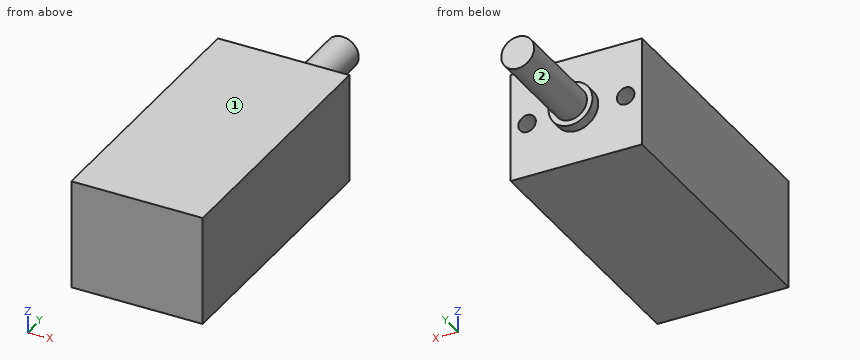
from build123d import *

# Parameters (mm, degrees)
SKETCH_1_W          = 12
SKETCH_1_H          = 10
EXTRUDE_1_DEPTH     = 25
SKETCH_2_R          = 2
EXTRUDE_2_DEPTH     = 1
SKETCH_3_R          = 1.5
EXTRUDE_3_DEPTH     = 9
SKETCH_4_R          = 0.8
CUT_EXTRUDE_1_DEPTH = 5


with BuildPart() as part:
    # 草图1 → 凸台-拉伸1 (new body)
    with BuildSketch(Plane(origin=(0, 0, 0), x_dir=(1, 0, 0), z_dir=(0, 1, 0))):
        Rectangle(SKETCH_1_W, SKETCH_1_H)
    extrude(amount=EXTRUDE_1_DEPTH)

    # 草图2 → 凸台-拉伸2 (add)
    with BuildSketch(Plane(origin=(0, 25, 0), x_dir=(1, 0, 0), z_dir=(0, 1, 0))):
        with Locations(Location((0, 0, 0), (0, 0, 270))):
            Circle(SKETCH_2_R)
    extrude(amount=EXTRUDE_2_DEPTH)

    # 草图3 → 凸台-拉伸3 (add)
    with BuildSketch(Plane(origin=(0, 26, 0), x_dir=(1, 0, 0), z_dir=(0, 1, 0))):
        with Locations(Location((0, 0, 0), (0, 0, 270))):
            Circle(SKETCH_3_R)
    extrude(amount=EXTRUDE_3_DEPTH)

    # 草图4 → 切除-拉伸1 (cut)
    with BuildSketch(Plane(origin=(0, 25, 0), x_dir=(1, 0, 0), z_dir=(0, 1, 0))):
        with Locations(Location((-4.5, 0, 0), (0, 0, 270))):
            Circle(SKETCH_4_R)
        with Locations(Location((4.5, 0, 0), (0, 0, 270))):
            Circle(SKETCH_4_R)
    extrude(amount=-CUT_EXTRUDE_1_DEPTH, mode=Mode.SUBTRACT)


solid = part.part
Can you work these out from the model? Positions are in its coordinate system, mm. Face numbers are marked on the shaded views. A direction names the side the tool comes from. Coordinates: 2 decimals unless noted, no trailing zeros. Write each loop counter-clockwise with the first axis right and the second up, starting at its lowest first coordinate (ties: lowest second). Pieces come first, ordered by that corner, then holes. Notation, with made-up numbers: (44.25, 70) - (56.25, 70) arc R22 cw to (56.25, 80) - close; hole circle Ø3 at (36, 34.5). An arc over 180 degrees is marked (long way). Return JSON: item names as keys, results as strings. Group by question number.
Item 1: If we section it at A-A (y = 20.5): Write out the boundary of the cut face in (x, z).
Item 2: I'm going to push flat-ended pins straight in: pin 1 Ø2 at (x, z) = (3.5, -2) entering from +Y; pin 2 Ø5 at (y, z) = (30, 1.5) entering from +X; pin 3 Ø0.8 at (x, z) = (-4.5, 0) entering from +Y. Where does each tip first touch, or does it pass through?
Item 3: Which directions (+Z, -Z, +X, -X, +Y, -Y) give clear straight access to the entire face, cutting with the end or side of a thin tool? Please do the marked faces 1 and 2.
Item 4: If we section it at D-D (y = 29.5): Write out the boundary of the cut face in (x, z), then the cut area to 3 significant figures.
Item 5: If we section it at B-B (x = 0): Write out the boundary of the cut face in (y, z), then the cut area to 3 significant figures.
Item 6: If we section it at C-C (z = 0): Write out the boundary of the cut face in (x, y), then the cut area to 3 significant figures.
Item 7: Please list where these lines run through material, in increasing order: probe 1 along X at (y, z) = (23.9, 0); probe 2 along Y at (x, z) = (4.25, 3.5); probe 3 along Y at (x, z) = (-4, 0.25).
Return value:
{
 "1": {"outline": "(-6, -5) - (6, -5) - (6, 5) - (-6, 5) - close; hole circle Ø1.6 at (-4.5, 0); hole circle Ø1.6 at (4.5, 0)"},
 "2": {"pin 1": "stops at y = 25", "pin 2": "stops at x = 1.5", "pin 3": "stops at y = 20"},
 "3": {"face 1": "+Z, +X, -X, +Y, -Y", "face 2": "+Y"},
 "4": {"outline": "circle Ø3 at (0, 0)", "area": "7.07 mm^2"},
 "5": {"outline": "(0, -5) - (25, -5) - (25, -2) - (26, -2) - (26, -1.5) - (35, -1.5) - (35, 1.5) - (26, 1.5) - (26, 2) - (25, 2) - (25, 5) - (0, 5) - close", "area": "281 mm^2"},
 "6": {"outline": "(-6, 0) - (6, 0) - (6, 25) - (5.3, 25) - (5.3, 20) - (3.7, 20) - (3.7, 25) - (2, 25) - (2, 26) - (1.5, 26) - (1.5, 35) - (-1.5, 35) - (-1.5, 26) - (-2, 26) - (-2, 25) - (-3.7, 25) - (-3.7, 20) - (-5.3, 20) - (-5.3, 25) - (-6, 25) - close", "area": "315 mm^2"},
 "7": {"probe 1": "x = -6 to -5.3, -3.7 to 3.7, 5.3 to 6", "probe 2": "y = 0 to 25", "probe 3": "y = 0 to 20"}
}
